from build123d import *

# Parameters (mm, degrees)
PAD_DEPTH     = 3
SKETCH001_R   = 14.5
SKETCH001_R_2 = 14
POCKET_DEPTH  = 3.001


with BuildPart() as part:
    # Sketch → Pad (new body)
    with BuildSketch(Plane.XY):
        Polygon((0, 495), (165, 495), (165, 0), (0, 0), (0, 247.5), align=None)
    extrude(amount=PAD_DEPTH)

    # Sketch001 (on Face7 of Pad) → Pocket (cut, through all)
    with BuildSketch(Plane.XY.offset(3)):
        with Locations((69.128997, 192.43482)):
            Circle(SKETCH001_R)
        with Locations((43.063397, 73.261589)):
            Circle(SKETCH001_R)
        with Locations((67.812135, 98.010326)):
            Circle(SKETCH001_R)
        with Locations((67.812135, 48.512852)):
            Circle(SKETCH001_R)
        with Locations((92.560872, 73.261589)):
            Circle(SKETCH001_R)
        with Locations((101.619539, 107.068993)):
            Circle(SKETCH001_R)
        with Locations((101.619539, 39.454185)):
            Circle(SKETCH001_R)
        with Locations((128.285753, 172.43482)):
            Circle(SKETCH001_R)
        with Locations((128.285753, 212.43482)):
            Circle(SKETCH001_R)
        with Locations((131.362427, 90.761589)):
            Circle(SKETCH001_R_2)
        with Locations((131.362427, 55.761589)):
            Circle(SKETCH001_R_2)
    extrude(amount=-POCKET_DEPTH, mode=Mode.SUBTRACT)


solid = part.part
Verification items for the finished model (mm, model axes). Give positions to 0.01 mm unless a question says otherwise; leave off trailing zeros. Write each loop counter-clockwise with the first axis right and the second up, starting at its lowest first coordinate (ties: lowest second). Pieces come first, ordered by that corner, then holes. Notation, with made-up numbers: (-36.75, 36) - (-1.75, 36) arc R20 ccw to (-1.75, 70) - close; hole circle Ø1 at (-9, 68.5). An arc over 180 degrees is marked (long way). Answer as CSV lines item,"result". Start each with the question number.
1. Sectioned sample at A-A (x = 41.5). Record the boundary of the cut face in (y, z).
2. Draft check along X on faces 1 (the face through (84, 251, 3)), 2 (the face through (115.45, 43.81, 1.52)), 3 (the face through (81.64, 52.87, 1.52)). Enter one of: pulls with the +X half, pulls with the -X half, needs draft (parallel to the pull), parting line crosses it, or undercut.
3. Sectioned sample at B-B (x = 134). Record the boundary of the cut face in (y, z), then the cut area to 3 significant figures.
4. Thickness scan on line 1 (Y direction, x = 69, z = 2.95); line 2 (Y direction, x = 117, z = 0.2); line 3 (Y direction, x = 112, z = 2.1). Record the ranges inside material, lowest first.
5. Sectioned sample at C-C (z = 0.45). Count the separate pieces of the cut face and the enclosed holes in it, then the cut area to 3 significant figures.
Derived:
1,outline,"(0, 0) - (58.85, 0) - (58.85, 3) - (0, 3) - close; (87.68, 0) - (495, 0) - (495, 3) - (87.68, 3) - close"
2,face 1,"needs draft"
2,face 2,"undercut"
2,face 3,"undercut"
3,outline,"(0, 0) - (42.01, 0) - (42.01, 3) - (0, 3) - close; (69.51, 0) - (77.01, 0) - (77.01, 3) - (69.51, 3) - close; (104.51, 0) - (159.11, 0) - (159.11, 3) - (104.51, 3) - close; (185.76, 0) - (199.11, 0) - (199.11, 3) - (185.76, 3) - close; (225.76, 0) - (495, 0) - (495, 3) - (225.76, 3) - close"
3,area,"1,160 mm²"
4,line 1,"0 to 34.06, 62.96 to 83.56, 112.46 to 177.94, 206.93 to 495"
4,line 2,"0 to 163.33, 181.54 to 203.33, 221.54 to 495"
4,line 3,"0 to 29.33, 49.58 to 96.94, 117.19 to 495"
5,separate pieces,"1"
5,enclosed holes,"11"
5,area,"74,500 mm²"
